from build123d import *

# Parameters (mm, degrees)
IZIM1_R                     = 3.1
IZIM1_R_2                   = 2.25
IZIM1_R_3                   = 2.5
Y_KSEKLIK_EKSTR_ZYON1_DEPTH = 5


with BuildPart() as part:
    # Çizim1 → Yükseklik-Ekstrüzyon1 (new body)
    with BuildSketch(Plane(origin=(0, 0, 0), x_dir=(1, 0, 0), z_dir=(0, 1, 0))):
        with BuildLine():
            Line((-39, 11.5), (-20, 11.5))
            ThreePointArc((-20, 11.5), (0, 31.5), (20, 11.5))
            Line((20, 11.5), (39, 11.5))
            Line((39, 11.5), (39, -11.5))
            Line((39, -11.5), (-39, -11.5))
            Line((-39, -11.5), (-39, 11.5))
        make_face()
        with Locations(Location((0, 23, 0), (0, 0, 270))):
            Circle(IZIM1_R, mode=Mode.SUBTRACT)
        with Locations(Location((-24.5, 6.5, 0), (0, 0, 270))):
            Circle(IZIM1_R_2, mode=Mode.SUBTRACT)
        with Locations(Location((-33, -5, 0), (0, 0, 270))):
            Circle(IZIM1_R_3, mode=Mode.SUBTRACT)
        with Locations(Location((33, -5, 0), (0, 0, 90))):
            Circle(IZIM1_R_3, mode=Mode.SUBTRACT)
        with Locations(Location((24.5, 6.5, 0), (0, 0, 90))):
            Circle(IZIM1_R_2, mode=Mode.SUBTRACT)
    extrude(amount=Y_KSEKLIK_EKSTR_ZYON1_DEPTH)


solid = part.part
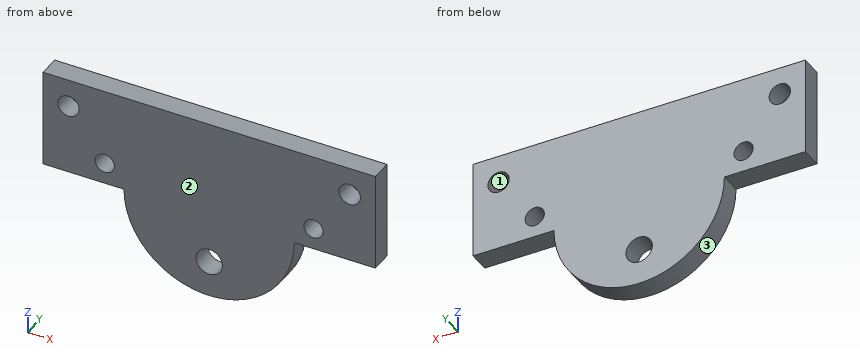
Model file for the job. Use its own axes, mm. Face numbers are marked on the shaded views. Give positions to 0.01 mm unless a question says otherwise; leave off trailing zeros. Write each loop counter-clockwise with the first axis right and the second up, starting at its lowest first coordinate (ties: lowest second). Pieces come first, ordered by that corner, then holes. Notation, with made-up numbers: (-19, -17.75) -> (4, -17.75) arc R16 cw to (4, 0.25) -> close; hole circle Ø1 at (61, -15). An arc over 180 degrees is marked (long way). Write item = value, one per line.
(1) Slice it at B-B, the plane x = -24.5. Give the cut face in (y, z).
Determined:
outline = (0, -11.5) -> (5, -11.5) -> (5, -8.75) -> (0, -8.75) -> close; (0, -4.25) -> (5, -4.25) -> (5, 11.5) -> (0, 11.5) -> close
(2) Flat gauge pins, fed straight in: P1, Ø12, axis at x = 27.5, z = -18.5, coming from the -Y side; P2, Ø1, axis at x = -9, y = 3, coming from the -Z side; P3, Ø1.5, axis at y = 1, z = -17, coming from the +X side. Where does each tip first touch, or does it go through?
Determined:
P1 = through
P2 = -29.6
P3 = 19.43
(3) Slice it at C-C, the plane y = 3.2. Give the cut face in (x, z).
Determined:
outline = (-39, -11.5) -> (-20, -11.5) arc R20 ccw to (20, -11.5) -> (39, -11.5) -> (39, 11.5) -> (-39, 11.5) -> close; hole circle Ø5 at (-33, 5); hole circle Ø4.5 at (-24.5, -6.5); hole circle Ø6.2 at (0, -23); hole circle Ø4.5 at (24.5, -6.5); hole circle Ø5 at (33, 5)
(4) Slice it at A-A, the plane z = 5. Give the cut face in (x, y).
Determined:
outline = (-39, 0) -> (-35.5, 0) -> (-35.5, 5) -> (-39, 5) -> close; (-30.5, 0) -> (30.5, 0) -> (30.5, 5) -> (-30.5, 5) -> close; (35.5, 0) -> (39, 0) -> (39, 5) -> (35.5, 5) -> close
(5) Slice it at D-D, the plane z = -23. Give the cut face in (x, y).
Determined:
outline = (-16.36, 0) -> (-3.1, 0) -> (-3.1, 5) -> (-16.36, 5) -> close; (3.1, 0) -> (16.36, 0) -> (16.36, 5) -> (3.1, 5) -> close
(6) Mould opens along Z. For the marked faces 1, 2 and 3 say: released by +Z, released by -Z, zero draft, split by the parting line, or undercut.
Determined:
face_1 = undercut
face_2 = zero draft
face_3 = released by -Z
(7) Probe line 1 along X through (y, z) = (3.7, 5); line 2 along Z through (x, y) = (24.5, 2.8); line 3 along X through (y, z) = (4.2, -8). List the from-to ranges inside material, lowest first.
Determined:
line_1 = -39 to -35.5, -30.5 to 30.5, 35.5 to 39
line_2 = -11.5 to -8.75, -4.25 to 11.5
line_3 = -39 to -26.18, -22.82 to 22.82, 26.18 to 39
